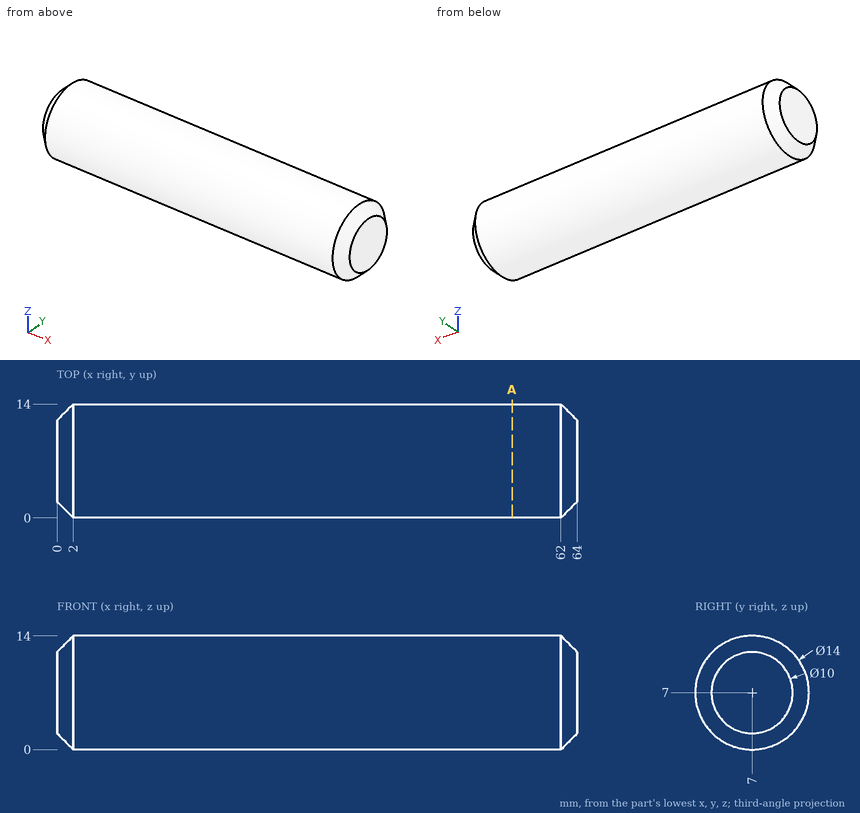
For this review, use the dimensioned drawing (mm, ordinates from the lowest corner) and the shaded views. Give positions to 0.01 mm unless a question says otherwise; leave off trailing zeros. Order: outer loops, then holes, each group sorted by start corner. A loop starts at its lowest first (then second) coordinate and runs counter-clockwise, first axis right, second up. Notation, with made-up numbers: (46.5, 57.5) -> (82.5, 57.5) arc R21 ccw to (82.5, 66.5) -> close; hole circle Ø4 at (45, 79). An arc over 180 degrees is marked (long way). Write item = value, one per line. Start each with the question number.
(1) For L1, parallel to Z at x = 51, y = 4; L2, parallel to X at y = 10, z = 1; L3, parallel to Y at x = 16.5, z = 11.75, list the stretches that pass through material, from the lowest coordinate up. Write a range as from..to.
(2) Take a section at A-A (x = 56). Write out the cut boundary in (y, z), plus the area to 3 significant figures.
(3) For pin 1 Ø4 at (x, y) = (8, 12) entering from +Z; pin 2 Ø1.5 at (x, y) = (31.5, 11) entering from +Z, all flat-tipped, find the tip position at first contact; note any pin that passes through.
Returned:
q1.L1 = 0.68..13.32
q1.L2 = 1.71..62.29
q1.L3 = 1.86..12.14
q2.outline = circle Ø14 at (7, 7)
q2.area = 154 mm²
q3.pin_1 = 13.32
q3.pin_2 = 13.2
